Input: part model. Units: mm. Frame: model coordinates. Face numbers are marked on the shaded views. A direction names the side the tool comes from. Give positions to 0.01 mm unless a question says otherwise; leave off trailing zeros. Order: outer loops, then holes, each group sorted by start corner. A loop starts at its lowest first (then second) coordinate and runs counter-clockwise, first axis right, second up. Notation, with made-up numbers: (0, 87.25) - (45, 87.25) arc R20 ccw to (45, 95.25) - close; hole circle Ø6 at (37, 14.25). An arc over 180 degrees is marked (long way). Answer in a Markdown table with one row per item. Add a question column.
1. Ray query, line 1 (X direction, y = 1.25, z = -26.5); line 2 (Y direction, x = 8.5, z = -20.5); line 3 (Z direction, x = -17, y = -8). Return the intervals inside material, ascending. Write a range as [from, to].
2. Section query D-D on y = -16. Return loops of the section in (x, z).
3. Section query B-B on x = -10. Return loops of the section in (y, z), and give its area (3 significant figures).
4. Section query A-A on y = -6.5. Count the separate pieces of the cut face and the enclosed holes in it, and give its area (3 significant figures).
5. Access query for the marked faces 1 and 2. Directions: +Z, -Z, +X, -X, +Y, -Y. A direction counts if a zero-diameter tool reaches every point of the face in a straight line with its end or side. Return the directions, or none.
6. Contact query for flat-ended pins moving along their axis: pin 1 (1.5 mm diameter, centred on y = -5, z = 1, fed in from +X); pin 2 (1.3 mm diameter, centred on x = 25, z = -3, fed in from -Y); pin 3 (1.2 mm diameter, centred on y = -1, z = -9, fed in from -X). Output: stop coordinate, or through.
7. Section query C-C on z = -21. Return loops of the section in (x, y).
8. Mould query, pull axis X, two halves, no side actions, for the marked faces 3, 4, 5 and 6. Classes: released by +X, released by -X, zero draft, split by the parting line, or undercut.
```python
from build123d import *

# Parameters (mm, degrees)
SKETCH1_W             = 60
SKETCH1_H             = 58
BOSS_EXTRUDE1_DEPTH   = 1.6
FILLET1_R             = 2
SKETCH2_R             = 1.5
CUT_EXTRUDE1_DEPTH    = 1.6
SKETCH3_R             = 6.25
BOSS_EXTRUDE2_DEPTH   = 20
SKETCH4_W             = 5
SKETCH4_H             = 30
BOSS_EXTRUDE3_DEPTH   = 10
SKETCH5_W             = 2.54
SKETCH5_H             = 2.54
BOSS_EXTRUDE4_DEPTH   = 2
FILLET2_R             = 0.5
SKETCH6_R             = 0.5
BOSS_EXTRUDE5_DEPTH   = 7
LPATTERN1_START       = -2
LPATTERN1_DEPTH       = 2
LPATTERN1_START_2     = -9
LPATTERN1_2_OUTLINE_R = 0.5
LPATTERN1_2_DEPTH     = 7


# Read off the part's stored shape, not the designer's step: LPattern1
with BuildPart() as part:
    # Sketch1 → Boss-Extrude1 (new body)
    with BuildSketch(Plane(origin=(0, 0, 0), x_dir=(1, 0, 0), z_dir=(0, 1, 0))):
        Rectangle(SKETCH1_W, SKETCH1_H)
    extrude(amount=BOSS_EXTRUDE1_DEPTH)

    # Fillet1
    fillet1_edges = [part.edges().sort_by_distance(p)[0] for p in [
        (-30, 0.8, -29),
        (30, 0.8, -29),
        (30, 0.8, 29),
        (-30, 0.8, 29),
    ]]
    fillet(fillet1_edges, radius=FILLET1_R)

    # Sketch2 → Cut-Extrude1 (cut)
    with BuildSketch(Plane.XZ):
        with Locations(Location((-27.5, 26.5, 0), (0, 0, 270))):
            Circle(SKETCH2_R)
        with Locations(Location((-27.5, -26.5, 0), (0, 0, 90))):
            Circle(SKETCH2_R)
        with Locations(Location((27.5, -26.5, 0), (0, 0, 270))):
            Circle(SKETCH2_R)
        with Locations(Location((27.5, 26.5, 0), (0, 0, 90))):
            Circle(SKETCH2_R)
    extrude(amount=-CUT_EXTRUDE1_DEPTH, mode=Mode.SUBTRACT)

    # Sketch3 → Boss-Extrude2 (add)
    with BuildSketch(Plane.XZ):
        with Locations(Location((-15, 19, 0), (0, 0, 90))):
            Circle(SKETCH3_R)
    extrude(amount=BOSS_EXTRUDE2_DEPTH)

    # Sketch4 → Boss-Extrude3 (add)
    with BuildSketch(Plane.XZ):
        with Locations((-24, -1)):
            Rectangle(SKETCH4_W, SKETCH4_H)
    extrude(amount=BOSS_EXTRUDE3_DEPTH)

    # Sketch5 → Boss-Extrude4 (add)
    with BuildSketch(Plane.XZ):
        with Locations((25, -19)):
            Rectangle(SKETCH5_W, SKETCH5_H)
    extrude(amount=BOSS_EXTRUDE4_DEPTH)

    # Fillet2
    fillet2_edges = [part.edges().sort_by_distance(p)[0] for p in [
        (26.27, -1, -20.27),
        (26.27, -1, -17.73),
        (23.73, -1, -17.73),
        (23.73, -1, -20.27),
    ]]
    fillet(fillet2_edges, radius=FILLET2_R)

    # Sketch6 → Boss-Extrude5 (add)
    with BuildSketch(Plane.XZ.offset(2)):
        with Locations(Location((25, -19, 0), (0, 0, 90))):
            Circle(SKETCH6_R)
    extrude(amount=BOSS_EXTRUDE5_DEPTH)

    # LPattern1 outline → LPattern1 (add)
    with BuildSketch(Plane(origin=(0, 0, 0), x_dir=(1, 0, 0), z_dir=(0, 1, 0)).offset(LPATTERN1_START)):
        with BuildLine():
            Line((26.27, 15.69), (26.27, 17.23))
            ThreePointArc((26.27, 17.23), (26.123553391, 17.583553391), (25.77, 17.73))
            Line((25.77, 17.73), (24.23, 17.73))
            ThreePointArc((24.23, 17.73), (23.876446609, 17.583553391), (23.73, 17.23))
            Line((23.73, 17.23), (23.73, 15.69))
            ThreePointArc((23.73, 15.69), (23.876446609, 15.336446609), (24.23, 15.19))
            ThreePointArc((24.23, 15.19), (23.876446609, 15.043553391), (23.73, 14.69))
            Line((23.73, 14.69), (23.73, 13.15))
            ThreePointArc((23.73, 13.15), (23.876446609, 12.796446609), (24.23, 12.65))
            ThreePointArc((24.23, 12.65), (23.876446609, 12.503553391), (23.73, 12.15))
            Line((23.73, 12.15), (23.73, 10.61))
            ThreePointArc((23.73, 10.61), (23.876446609, 10.256446609), (24.23, 10.11))
            ThreePointArc((24.23, 10.11), (23.876446609, 9.963553391), (23.73, 9.61))
            Line((23.73, 9.61), (23.73, 8.07))
            ThreePointArc((23.73, 8.07), (23.876446609, 7.716446609), (24.23, 7.57))
            ThreePointArc((24.23, 7.57), (23.876446609, 7.423553391), (23.73, 7.07))
            Line((23.73, 7.07), (23.73, 5.53))
            ThreePointArc((23.73, 5.53), (23.876446609, 5.176446609), (24.23, 5.03))
            ThreePointArc((24.23, 5.03), (23.876446609, 4.883553391), (23.73, 4.53))
            Line((23.73, 4.53), (23.73, 2.99))
            ThreePointArc((23.73, 2.99), (23.876446609, 2.636446609), (24.23, 2.49))
            ThreePointArc((24.23, 2.49), (23.876446609, 2.343553391), (23.73, 1.99))
            Line((23.73, 1.99), (23.73, 0.45))
            ThreePointArc((23.73, 0.45), (23.876446609, 0.096446609), (24.23, -0.05))
            ThreePointArc((24.23, -0.05), (23.876446609, -0.196446609), (23.73, -0.55))
            Line((23.73, -0.55), (23.73, -2.09))
            ThreePointArc((23.73, -2.09), (23.876446609, -2.443553391), (24.23, -2.59))
            ThreePointArc((24.23, -2.59), (23.876446609, -2.736446609), (23.73, -3.09))
            Line((23.73, -3.09), (23.73, -4.63))
            ThreePointArc((23.73, -4.63), (23.876446609, -4.983553391), (24.23, -5.13))
            ThreePointArc((24.23, -5.13), (23.876446609, -5.276446609), (23.73, -5.63))
            Line((23.73, -5.63), (23.73, -7.17))
            ThreePointArc((23.73, -7.17), (23.876446609, -7.523553391), (24.23, -7.67))
            ThreePointArc((24.23, -7.67), (23.876446609, -7.816446609), (23.73, -8.17))
            Line((23.73, -8.17), (23.73, -9.71))
            ThreePointArc((23.73, -9.71), (23.876446609, -10.063553391), (24.23, -10.21))
            ThreePointArc((24.23, -10.21), (23.876446609, -10.356446609), (23.73, -10.71))
            Line((23.73, -10.71), (23.73, -12.25))
            ThreePointArc((23.73, -12.25), (23.876446609, -12.603553391), (24.23, -12.75))
            Line((24.23, -12.75), (25.77, -12.75))
            ThreePointArc((25.77, -12.75), (26.123553391, -12.603553391), (26.27, -12.25))
            Line((26.27, -12.25), (26.27, -10.71))
            ThreePointArc((26.27, -10.71), (26.123553391, -10.356446609), (25.77, -10.21))
            ThreePointArc((25.77, -10.21), (26.123553391, -10.063553391), (26.27, -9.71))
            Line((26.27, -9.71), (26.27, -8.17))
            ThreePointArc((26.27, -8.17), (26.123553391, -7.816446609), (25.77, -7.67))
            ThreePointArc((25.77, -7.67), (26.123553391, -7.523553391), (26.27, -7.17))
            Line((26.27, -7.17), (26.27, -5.63))
            ThreePointArc((26.27, -5.63), (26.123553391, -5.276446609), (25.77, -5.13))
            ThreePointArc((25.77, -5.13), (26.123553391, -4.983553391), (26.27, -4.63))
            Line((26.27, -4.63), (26.27, -3.09))
            ThreePointArc((26.27, -3.09), (26.123553391, -2.736446609), (25.77, -2.59))
            ThreePointArc((25.77, -2.59), (26.123553391, -2.443553391), (26.27, -2.09))
            Line((26.27, -2.09), (26.27, -0.55))
            ThreePointArc((26.27, -0.55), (26.123553391, -0.196446609), (25.77, -0.05))
            ThreePointArc((25.77, -0.05), (26.123553391, 0.096446609), (26.27, 0.45))
            Line((26.27, 0.45), (26.27, 1.99))
            ThreePointArc((26.27, 1.99), (26.123553391, 2.343553391), (25.77, 2.49))
            ThreePointArc((25.77, 2.49), (26.123553391, 2.636446609), (26.27, 2.99))
            Line((26.27, 2.99), (26.27, 4.53))
            ThreePointArc((26.27, 4.53), (26.123553391, 4.883553391), (25.77, 5.03))
            ThreePointArc((25.77, 5.03), (26.123553391, 5.176446609), (26.27, 5.53))
            Line((26.27, 5.53), (26.27, 7.07))
            ThreePointArc((26.27, 7.07), (26.123553391, 7.423553391), (25.77, 7.57))
            ThreePointArc((25.77, 7.57), (26.123553391, 7.716446609), (26.27, 8.07))
            Line((26.27, 8.07), (26.27, 9.61))
            ThreePointArc((26.27, 9.61), (26.123553391, 9.963553391), (25.77, 10.11))
            ThreePointArc((25.77, 10.11), (26.123553391, 10.256446609), (26.27, 10.61))
            Line((26.27, 10.61), (26.27, 12.15))
            ThreePointArc((26.27, 12.15), (26.123553391, 12.503553391), (25.77, 12.65))
            ThreePointArc((25.77, 12.65), (26.123553391, 12.796446609), (26.27, 13.15))
            Line((26.27, 13.15), (26.27, 14.69))
            ThreePointArc((26.27, 14.69), (26.123553391, 15.043553391), (25.77, 15.19))
            ThreePointArc((25.77, 15.19), (26.123553391, 15.336446609), (26.27, 15.69))
        make_face()
    extrude(amount=LPATTERN1_DEPTH)

    # LPattern1 2 outline → LPattern1 2 (add)
    with BuildSketch(Plane(origin=(0, 0, 0), x_dir=(1, 0, 0), z_dir=(0, 1, 0)).offset(LPATTERN1_START_2)):
        with Locations((25, 16.46)):
            Circle(LPATTERN1_2_OUTLINE_R)
        with Locations((25, 13.92)):
            Circle(LPATTERN1_2_OUTLINE_R)
        with Locations((25, 11.38)):
            Circle(LPATTERN1_2_OUTLINE_R)
        with Locations((25, 8.84)):
            Circle(LPATTERN1_2_OUTLINE_R)
        with Locations((25, 6.3)):
            Circle(LPATTERN1_2_OUTLINE_R)
        with Locations((25, 3.76)):
            Circle(LPATTERN1_2_OUTLINE_R)
        with Locations((25, 1.22)):
            Circle(LPATTERN1_2_OUTLINE_R)
        with Locations((25, -1.32)):
            Circle(LPATTERN1_2_OUTLINE_R)
        with Locations((25, -3.86)):
            Circle(LPATTERN1_2_OUTLINE_R)
        with Locations((25, -6.4)):
            Circle(LPATTERN1_2_OUTLINE_R)
        with Locations((25, -8.94)):
            Circle(LPATTERN1_2_OUTLINE_R)
        with Locations((25, -11.48)):
            Circle(LPATTERN1_2_OUTLINE_R)
    extrude(amount=LPATTERN1_2_DEPTH)


solid = part.part
```
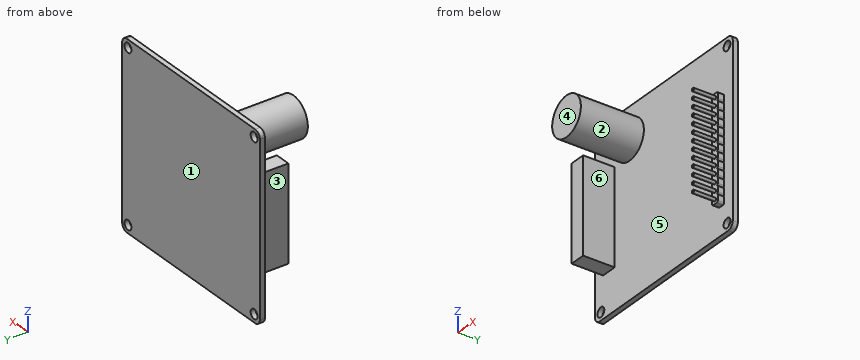
Answer:
| question | item | result |
|---|---|---|
| 1 | line 1 | x = [-30, -29], [-26, 26], [29, 30] |
| 1 | line 2 | y = [0, 1.6] |
| 1 | line 3 | z = [13.08, 24.92] |
| 2 | outline | circle Ø12.5 at (-15, 19) |
| 3 | outline | (-20, 15.25) - (0, 15.25) - (0, -29) - (1.6, -29) - (1.6, 29) - (0, 29) - (0, 22.75) - (-20, 22.75) - close |
| 3 | area | 243 mm² |
| 4 | separate pieces | 15 |
| 4 | enclosed holes | 0 |
| 4 | area | 283 mm² |
| 5 | face 1 | +Z, -Z, +X, -X, +Y |
| 5 | face 2 | -Y |
| 6 | pin 1 | stops at x = 25.5 |
| 6 | pin 2 | stops at y = -9 |
| 6 | pin 3 | stops at x = -26.5 |
| 7 | outline | (-30, 0) - (30, 0) - (30, 1.6) - (-30, 1.6) - close |
| 8 | face 3 | released by -X |
| 8 | face 4 | zero draft |
| 8 | face 5 | undercut |
| 8 | face 6 | undercut |
